from build123d import *

# Parameters (mm, degrees)
BOSS_EXTRUDE1_DEPTH          = 25.4
F_3_0_3_DIAMETER_HOLE1_D     = 3
F_3_0_3_DIAMETER_HOLE1_DEPTH = 25.4
CHAMFER1_SIZE                = 0.35


with BuildPart() as part:
    # Sketch1 → Boss-Extrude1 (new body)
    with BuildSketch(Plane.XY.offset(25.4)):
        Polygon((-3.579571669, 0), (-1.789785834, -3.1), (1.789785834, -3.1), (3.579571669, 0), (1.789785834, 3.1), (-1.789785834, 3.1), align=None)
    extrude(amount=-BOSS_EXTRUDE1_DEPTH)

    # Ø3.0 (3) Diameter Hole1
    with Locations(Plane.XY.offset(25.4)):
        with Locations((0, 0)):
            Hole(F_3_0_3_DIAMETER_HOLE1_D / 2, depth=F_3_0_3_DIAMETER_HOLE1_DEPTH)

    # Chamfer1
    chamfer1_edges = [part.edges().sort_by_distance(p)[0] for p in [
        (1.5, 0, 25.4),
        (1.5, 0, 0),
    ]]
    chamfer(chamfer1_edges, length=CHAMFER1_SIZE)


solid = part.part
Source: CAD feature listing. Evaluate the final solid. Frame: model axes, mm. Coordinates: 2 decimals unless noted, no trailing zeros. Loops run counter-clockwise (first coordinate to the right, second up) from the corner with the lowest first, then second, coordinate; pieces in that order, holes last. Notation, with made-up numbers: (-2, 88.5) - (12, 88.5) arc R11 cw to (12, 105.5) - close; hole circle Ø7 at (24, -27). An arc over 180 degrees is marked (long way). Return JSON: item names as keys, results as strings.
Q1. Mould query, pull axis Y, two halves, no side actions, for faces 1 (the cylindrical face through (1.5, 0.07, 12.53)), 2 (the flat face through (2, 1, 25.4)), 3 (the flat face through (0, -3.1, 13)). Classes: released by +Y, released by -Y, zero draft, split by the parting line, or undercut.
Results:
{"face 1": "undercut", "face 2": "zero draft", "face 3": "released by -Y"}
Q2. Section D-D, the plane x = 2.75. Return loops of the section in (y, z), plus the area to 3 significant figures.
Results:
{"outline": "(-1.44, 0) - (1.44, 0) - (1.44, 25.4) - (-1.44, 25.4) - close", "area": "73.0 mm2"}
Q3. Section C-C, the plane y = -2.25. Return loops of the section in (x, z).
Results:
{"outline": "(-2.28, 0) - (2.28, 0) - (2.28, 25.4) - (-2.28, 25.4) - close"}
Q4. Section A-A, the plane x = 0. Return loops of the section in (y, z).
Results:
{"outline": "(-3.1, 0) - (-1.85, 0) - (-1.5, 0.35) - (-1.5, 25.05) - (-1.85, 25.4) - (-3.1, 25.4) - close; (1.5, 0.35) - (1.85, 0) - (3.1, 0) - (3.1, 25.4) - (1.85, 25.4) - (1.5, 25.05) - close"}
Q5. Section B-B, the plane z = 2.75. Return loops of the section in (x, y).
Results:
{"outline": "(-3.58, 0) - (-1.79, -3.1) - (1.79, -3.1) - (3.58, 0) - (1.79, 3.1) - (-1.79, 3.1) - close; hole circle Ø3 at (0, 0)"}
Q6. Contact query for flat-ended pins moving along their axis: P1, Ø3.5, axis at x = 0, y = 0, coming from the +Z side; P2, Ø2, axis at y = -2, z = 21, coming from the -X side. Output: stop coordinate, or through.
Results:
{"P1": "z = 25.3", "P2": "x = -3"}
Q7. Material intervals for line 1 along Y through (x, z) = (0, 20); line 2 along X through (y, z) = (1, 14.5); line 3 along X through (y, z) = (-0.5, 1.5), sorted ascending.
Results:
{"line 1": "-3.1 to -1.5, 1.5 to 3.1", "line 2": "-3 to -1.12, 1.12 to 3", "line 3": "-3.29 to -1.41, 1.41 to 3.29"}
